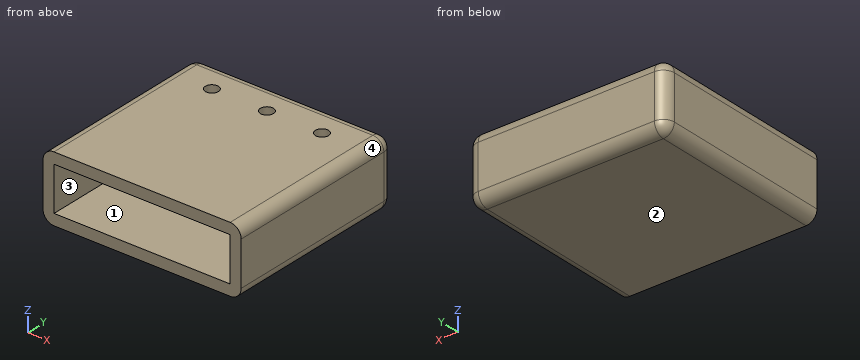
Autodesk Fusion 360 part; units mm, degrees
sketch "Skizze1" plane through (0, 0, 0) normal (0, 0, 1) x (1, 0, 0)
  line L0 (-50, 50) -> (40, 50)
  line L1 (40, 50) -> (40, -35)
  line L2 (40, -35) -> (-50, -35)
  line L3 (-50, -35) -> (-50, 50)
  dimension "d1" = 90
  dimension "d2" = 85
extrude "Extrusion1" add sketch "Skizze1" along normal blind 30
shell "Schale1" thickness 5 removed faces 1 at (10, -35, 20)
fillet "Abrundung1" radius 5 1 edges at (-5, 50, 30)
fillet "Abrundung2" radius 5 3 edges at (40, 5, 30) (40, 48.5355, 28.5355) (40, 50, 12.5)
fillet "Abrundung3" radius 5 3 edges at (-50, 50, 12.5) (-50, 48.5355, 28.5355) (-50, 5, 30)
fillet "Abrundung4" radius 5 5 edges at (-50, 5, 0) (-48.5355, 48.5355, 0) (-5, 50, 0) (38.5355, 48.5355, 0) (40, 5, 0)
sketch "Skizze2" plane through (0, 0, 30) normal (0, 0, 1) x (-1, 0, 0)
  line L0 (45, -45) -> (45, 35)
  line L1 (45, 35) -> (-35, 35)
  line L2 (-35, 35) -> (-35, -45)
  line L3 (-35, -45) -> (45, -45)
  circle A0 centre (5, -35) radius 3
  circle A1 centre (30, -35) radius 3
  circle A2 centre (-20, -35) radius 3
extrude "Extrusion2" cut sketch "Skizze2" along normal mid plane 10 contours A1
extrude "Extrusion3" cut sketch "Skizze2" along normal mid plane 10 contours A0 | A2
The model under review builds one solid part; all positions refer to its coordinate system, in mm. Face numbers are marked on the shaded views. Round coordinates to 2 decimals unless told otherwise and drop trailing zeros. Order: outer loops, then holes, each group sorted by start corner. A loop starts at its lowest first (then second) coordinate and runs counter-clockwise, first axis right, second up. Notation, with made-up numbers: (14, 66) - (33, 66) arc R26 cw to (33, 101) - close; hole circle Ø7 at (41, 10.5). An arc over 180 degrees is marked (long way). Answer in a Markdown table with one row per item.
(1) Mouldability with a two-part tool opening along X and no side actions: class the marked faces 1, 2, 3 and 4 as released by +X, released by -X, zero draft, split by the parting line, or undercut.
Result set:
| item | result |
|---|---|
| face 1 | undercut |
| face 2 | zero draft |
| face 3 | undercut |
| face 4 | released by +X |
(2) For line 1 (X direction, y = 12, z = 5.5); line 2 (Z direction, x = 2, y = 17.5); line 3 (X direction, y = 35, z = 28.3), list the stretches that pass through material, from the lowest coordinate up. Write a range as from..to.
Result set:
| item | result |
|---|---|
| line 1 | x = -50..-45, 35..40 |
| line 2 | z = 0..5, 25..30 |
| line 3 | x = -48.76..-33, -27..-8, -2..17, 23..38.76 |
(3) Take a section at B-B on y = 35. Write out the cut boundary in (x, z), plus the area to 3 significant figures.
Result set:
| item | result |
|---|---|
| outline | (-50, 5) arc R5 ccw to (-45, 0) - (35, 0) arc R5 ccw to (40, 5) - (40, 25) arc R5 ccw to (35, 30) - (23, 30) - (23, 25) - (35, 25) - (35, 5) - (-45, 5) - (-45, 25) - (-33, 25) - (-33, 30) - (-45, 30) arc R5 ccw to (-50, 25) - close; (-27, 25) - (-8, 25) - (-8, 30) - (-27, 30) - close; (-2, 25) - (17, 25) - (17, 30) - (-2, 30) - close |
| area | 989 mm2 |
(4) Clearance check with flat-ended pins moving along their axes: P1, Ø6, axis at x = -5.5, z = 18.5, coming from the -Y side; P2, Ø1.5, axis at x = 29.5, z = 24.5, coming from the -Y side; P3, Ø3.5, axis at x = -5, y = 35, coming from the +Z side. State where each tip first meets the part, or that it passes through.
Result set:
| item | result |
|---|---|
| P1 | stops at y = 45 |
| P2 | stops at y = -35 |
| P3 | stops at z = 5 |
(5) Take a section at A-A on x = -5. Write out the cut boundary in (y, z), plus the area to 3 significant figures.
Result set:
| item | result |
|---|---|
| outline | (-35, 0) - (45, 0) arc R5 ccw to (50, 5) - (50, 25) arc R5 ccw to (45, 30) - (38, 30) - (38, 25) - (45, 25) - (45, 5) - (-35, 5) - close; (-35, 25) - (32, 25) - (32, 30) - (-35, 30) - close |
| area | 909 mm2 |
(6) Take a section at D-D on x = 12.5. Write out the cut boundary in (y, z), plus the area to 3 significant figures.
Result set:
| item | result |
|---|---|
| outline | (-35, 0) - (45, 0) arc R5 ccw to (50, 5) - (50, 25) arc R5 ccw to (45, 30) - (-35, 30) - (-35, 25) - (45, 25) - (45, 5) - (-35, 5) - close |
| area | 939 mm2 |
(7) Take a section at C-C on z = 27.5. Write out the cut boundary in (x, y).
Result set:
| item | result |
|---|---|
| outline | (-49.33, -35) - (39.33, -35) - (39.33, 45) arc R4.33 ccw to (35, 49.33) - (-45, 49.33) arc R4.33 ccw to (-49.33, 45) - close; hole circle Ø6 at (-30, 35); hole circle Ø6 at (-5, 35); hole circle Ø6 at (20, 35) |
